Read the model definition and answer for the solid it produces. Units are mm, in the model's axes. Give positions to 0.01 mm unless a question says otherwise; leave off trailing zeros. Order: outer loops, then holes, each group sorted by start corner. A loop starts at its lowest first (then second) coordinate and runs counter-clockwise, first axis right, second up. Notation, with made-up numbers: (23.5, 75) - (51.5, 75) arc R18 cw to (51.5, 108) - close; hole circle Ø6 at (-12, -10.5). An arc over 180 degrees is marked (long way). One line per item, written item: value. Start each with the question number.
```python
from build123d import *

# Parameters (mm, degrees)
MODEL_W             = 5
MODEL_H             = 5.35
MODEL_W_2           = 14
MODEL_W_3           = 11
MODEL_W_4           = 5.35
MODEL_H_2           = 20
BOSS_EXTRUDE1_DEPTH = 5.35


with BuildPart() as part:
    # Model → Boss-Extrude1 (new body)
    with BuildSketch(Plane.XY):
        with BuildLine():
            Line((-55.695, 30), (-36.5, 30))
            ThreePointArc((-36.5, 30), (-35.439339828, 30.439339828), (-35, 31.5))
            Line((-35, 31.5), (-35, 200))
            Line((-35, 200), (35, 200))
            Line((35, 200), (35, 31.5))
            ThreePointArc((35, 31.5), (35.439339828, 30.439339828), (36.5, 30))
            Line((36.5, 30), (55.695, 30))
            ThreePointArc((55.695, 30), (57.109213562, 29.414213562), (57.695, 28))
            Line((57.695, 28), (57.695, 2))
            ThreePointArc((57.695, 2), (57.109213562, 0.585786438), (55.695, 0))
            Line((55.695, 0), (-55.695, 0))
            ThreePointArc((-55.695, 0), (-57.109213562, 0.585786438), (-57.695, 2))
            Line((-57.695, 2), (-57.695, 28))
            ThreePointArc((-57.695, 28), (-57.109213562, 29.414213562), (-55.695, 30))
        make_face()
        with Locations((53.175, 10.225)):
            Rectangle(MODEL_W, MODEL_H, mode=Mode.SUBTRACT)
        with Locations((-53.175, 10.225)):
            Rectangle(MODEL_W, MODEL_H, mode=Mode.SUBTRACT)
        with Locations((14.25, 42.025)):
            Rectangle(MODEL_W_2, MODEL_H, mode=Mode.SUBTRACT)
        with Locations((0, 145.75)):
            Rectangle(MODEL_W_3, MODEL_H, mode=Mode.SUBTRACT)
        with Locations((0, 104.25)):
            Rectangle(MODEL_W_3, MODEL_H, mode=Mode.SUBTRACT)
        with Locations((-14, 189.825)):
            Rectangle(MODEL_W_2, MODEL_H, mode=Mode.SUBTRACT)
        with Locations((-27.155, 167.5)):
            Rectangle(MODEL_W_4, MODEL_H_2, mode=Mode.SUBTRACT)
        with Locations((-27.155, 125)):
            Rectangle(MODEL_W_4, MODEL_H_2, mode=Mode.SUBTRACT)
        with Locations((-27.155, 82.5)):
            Rectangle(MODEL_W_4, MODEL_H_2, mode=Mode.SUBTRACT)
        with Locations((-14.25, 42.025)):
            Rectangle(MODEL_W_2, MODEL_H, mode=Mode.SUBTRACT)
        with Locations((27.155, 82.5)):
            Rectangle(MODEL_W_4, MODEL_H_2, mode=Mode.SUBTRACT)
        with Locations((27.155, 125)):
            Rectangle(MODEL_W_4, MODEL_H_2, mode=Mode.SUBTRACT)
        with Locations((27.155, 167.5)):
            Rectangle(MODEL_W_4, MODEL_H_2, mode=Mode.SUBTRACT)
        with Locations((14, 189.825)):
            Rectangle(MODEL_W_2, MODEL_H, mode=Mode.SUBTRACT)
        with Locations((-28.175, 10.225)):
            Rectangle(MODEL_W, MODEL_H, mode=Mode.SUBTRACT)
        with BuildLine():
            Line((-53.195, 26), (-44.195, 26))
            ThreePointArc((-44.195, 26), (-43.841446609, 25.853553391), (-43.695, 25.5))
            Line((-43.695, 25.5), (-43.695, 17.5))
            ThreePointArc((-43.695, 17.5), (-43.841446609, 17.146446609), (-44.195, 17))
            Line((-44.195, 17), (-53.195, 17))
            ThreePointArc((-53.195, 17), (-53.548553391, 17.146446609), (-53.695, 17.5))
            Line((-53.695, 17.5), (-53.695, 25.5))
            ThreePointArc((-53.695, 25.5), (-53.548553391, 25.853553391), (-53.195, 26))
        make_face(mode=Mode.SUBTRACT)
        with Locations((28.175, 10.225)):
            Rectangle(MODEL_W, MODEL_H, mode=Mode.SUBTRACT)
    extrude(amount=BOSS_EXTRUDE1_DEPTH)


solid = part.part
```
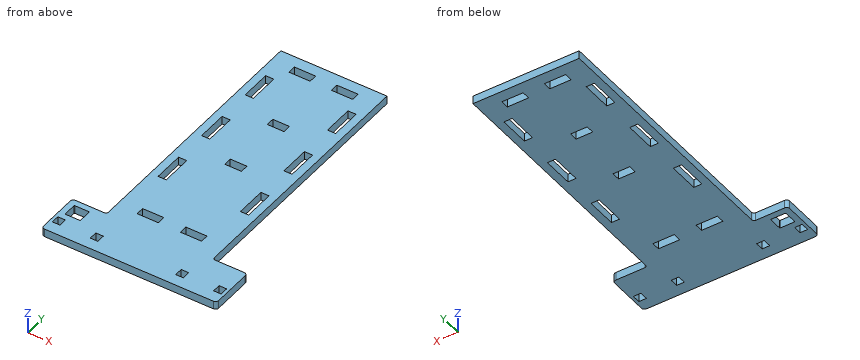
1) Find the intervals of material crossed by probe 1 along Y at (x, z) = (-28.5, 0.3); probe 2 along X at (y, z) = (82.5, 2.1); probe 3 along Y at (x, z) = (-3, 4.2) (3 decimals), in increasing order. Write a range as from..to.
2) Each of these flat-tipped pins is pushed along its axis until it touches: pin 1 (2.5 mm diameter, centred on y = 169, z = 2, fed in from -X); pin 2 (2 mm diameter, centred on x = -5.5, z = 3.5, fed in from -Y); pin 3 (1.6 mm diameter, centred on x = 42, z = 2, fed in from +Y); pin 4 (2.5 mm diameter, centred on y = 163, z = 2.5, fed in from +X). Where does it stop, or does it pass through?
3) Section A-A on y = 174 is taken. Write down the section's boundary in (x, z), plus the area to 3 significant figures.
4) Section B-B on x = 18 is taken. Write down the section's boundary in (y, z).
5) Section D-D on x = 41 is taken. Write down the section's boundary in (y, z).
6) Section C-C on y = 20 is taken. Write down the section's boundary in (x, z) (3 decimals).
Solved:
1. probe 1: y = 0..7.55, 12.9..72.5, 92.5..115, 135..157.5, 177.5..200
1. probe 2: x = -35..-29.83, -24.48..24.48, 29.83..35
1. probe 3: y = 0..101.575, 106.925..143.075, 148.425..200
2. pin 1: stops at x = -35
2. pin 2: stops at y = 0
2. pin 3: stops at y = 30
2. pin 4: stops at x = 35
3. outline: (-35, 0) - (-29.83, 0) - (-29.83, 5.35) - (-35, 5.35) - close; (-24.48, 0) - (24.48, 0) - (24.48, 5.35) - (-24.48, 5.35) - close; (29.83, 0) - (35, 0) - (35, 5.35) - (29.83, 5.35) - close
3. area: 317 mm2
4. outline: (0, 0) - (39.35, 0) - (39.35, 5.35) - (0, 5.35) - close; (44.7, 0) - (187.15, 0) - (187.15, 5.35) - (44.7, 5.35) - close; (192.5, 0) - (200, 0) - (200, 5.35) - (192.5, 5.35) - close
5. outline: (0, 0) - (30, 0) - (30, 5.35) - (0, 5.35) - close
6. outline: (-57.695, 0) - (-53.695, 0) - (-53.695, 5.35) - (-57.695, 5.35) - close; (-43.695, 0) - (57.695, 0) - (57.695, 5.35) - (-43.695, 5.35) - close
